Design review of the part built by this model. Coordinates are the model's own, in mm. A direction names the side the tool comes from. Round coordinates to 2 decimals unless told otherwise and drop trailing zeros. Loops run counter-clockwise (first coordinate to the right, second up) from the corner with the lowest first, then second, coordinate; pieces in that order, holes last. Notation, with made-up numbers: (56.5, 77) -> (72.5, 77) arc R22 ccw to (72.5, 102) -> close; hole circle Ø6 at (-27.75, 88.5). An arc over 180 degrees is marked (long way). Use a Markdown table: item, result. Add a question column.
from build123d import *

# Parameters (mm, degrees)
SKETCH1_W           = 50.8
SKETCH1_H           = 57.15
BOSS_EXTRUDE1_DEPTH = 6.35
SKETCH5_R           = 1.524
SKETCH5_R_2         = 2.54
CUT_EXTRUDE1_DEPTH  = 72.447438113
SKETCH6_W           = 4.7625
SKETCH6_H           = 2.38125
SKETCH6_W_2         = 4.700923451
CUT_EXTRUDE2_DEPTH  = 72.447438113
SKETCH7_W           = 50.8
SKETCH7_H           = 25.4
CUT_EXTRUDE3_DEPTH  = 72.447438113


with BuildPart() as part:
    # Sketch1 → Boss-Extrude1 (new body)
    with BuildSketch(Plane.XY):
        with Locations((-32.446072824, -12.876728212)):
            Rectangle(SKETCH1_W, SKETCH1_H)
    extrude(amount=BOSS_EXTRUDE1_DEPTH)

    # Sketch5 → Cut-Extrude1 (cut, through all)
    with BuildSketch(Plane.XY.offset(6.35)):
        with Locations((-11.808572824, -26.275228212)):
            Circle(SKETCH5_R)
        with Locations((-11.808572824, -36.689228212)):
            Circle(SKETCH5_R)
        with Locations((-34.160572824, -26.275228212)):
            Circle(SKETCH5_R)
        with Locations((-34.160572824, -36.689228212)):
            Circle(SKETCH5_R)
        with Locations((-48.321072824, 10.618271788)):
            Circle(SKETCH5_R_2)
        with Locations((-16.571072824, 10.618271788)):
            Circle(SKETCH5_R_2)
        with Locations((-48.321072824, -2.081728212)):
            Circle(SKETCH5_R_2)
        with Locations((-16.571072824, -2.081728212)):
            Circle(SKETCH5_R_2)
        with Locations((-48.321072824, -14.781728212)):
            Circle(SKETCH5_R_2)
        with Locations((-16.571072824, -14.781728212)):
            Circle(SKETCH5_R_2)
    extrude(amount=-CUT_EXTRUDE1_DEPTH, mode=Mode.SUBTRACT)

    # Sketch6 → Cut-Extrude2 (cut, through all)
    with BuildSketch(Plane.XY.offset(6.35)):
        with Locations((-52.289822824, -33.911103212)):
            Rectangle(SKETCH6_W, SKETCH6_H)
        with Locations((-52.320611099, -24.900183987)):
            Rectangle(SKETCH6_W_2, SKETCH6_H)
    extrude(amount=-CUT_EXTRUDE2_DEPTH, mode=Mode.SUBTRACT)

    # Sketch7 → Cut-Extrude3 (cut, through all)
    with BuildSketch(Plane.XY.offset(6.35)):
        with Locations((-32.446072824, 2.998271788)):
            Rectangle(SKETCH7_W, SKETCH7_H)
    extrude(amount=-CUT_EXTRUDE3_DEPTH, mode=Mode.SUBTRACT)


solid = part.part
1. Consider section C-C on y = -37.5. State the section outline as (x, z) points, plus the area to 3 significant figures.
2. Mouldability with a two-part tool opening along X and no side actions: class faces 3 (the face through (-49.909, -34, 3)), 4 (the face through (-33, -25, 0)), 5 (the face through (-54.671, -34, 3)), 6 (the face through (-7.046, -26, 3)) as +X half, -X half, draft (parallel to the pull), parting line (faces both ways), or undercut.
3. To check wall thickness, follow probe 1 along Y at (x, z) = (-52, 3); probe 2 along X at (y, z) = (-33.5, 4.75); probe 3 along X at (y, z) = (-16.5, 5.5). State the ranges of each line that lie inside material, in increasing order. Write a range as from..to.
4. Insertion check: P1, Ø1.8, axis at x = -11.81, y = -36.69, coming from the -Z side. The pin has a flat end and moves straight along its axis. Give the tip position at first contact, or say it passes through.
5. Consider section B-B on z = 4.75. Give the number of separate pieces and of enclosed holes in the cut face, plus the area to 3 significant figures.
6. Consider section A-A on y = -13. State the section outline as (x, z) points.
7. For faces 1 (the face through (-49.97, -25, 3)), 2 (the face through (-57.846, -26, 3)), list the 3-axis set-ups (+Z, -Z, +X, -X, +Y, -Y) from which the entire face can be reached by the end or side of a thin tool; tool diameter is ignored.
Verdict:
| question | item | result |
|---|---|---|
| 1 | outline | (-57.85, 0) -> (-35.45, 0) -> (-35.45, 6.35) -> (-57.85, 6.35) -> close; (-32.87, 0) -> (-13.1, 0) -> (-13.1, 6.35) -> (-32.87, 6.35) -> close; (-10.52, 0) -> (-7.05, 0) -> (-7.05, 6.35) -> (-10.52, 6.35) -> close |
| 1 | area | 290 mm² |
| 2 | face 3 | undercut |
| 2 | face 4 | draft |
| 2 | face 5 | undercut |
| 2 | face 6 | +X half |
| 3 | probe 1 | y = -41.45..-35.1, -32.72..-26.09, -23.71..-9.7 |
| 3 | probe 2 | x = -57.85..-54.67, -49.91..-7.05 |
| 3 | probe 3 | x = -57.85..-50.19, -46.45..-18.44, -14.7..-7.05 |
| 4 | P1 | passes through |
| 5 | separate pieces | 1 |
| 5 | enclosed holes | 8 |
| 5 | area | 1,520 mm² |
| 6 | outline | (-57.85, 0) -> (-50.13, 0) -> (-50.13, 6.35) -> (-57.85, 6.35) -> close; (-46.51, 0) -> (-18.38, 0) -> (-18.38, 6.35) -> (-46.51, 6.35) -> close; (-14.76, 0) -> (-7.05, 0) -> (-7.05, 6.35) -> (-14.76, 6.35) -> close |
| 7 | face 1 | +Z, -Z |
| 7 | face 2 | +Z, -Z, -X, +Y, -Y |
